Can you work these out from the model? Positions are in its coordinate system, mm. Face numbers are marked on the shaded views. A direction names the side the tool comes from. Give positions to 0.01 mm unless a question says otherwise; leave off trailing zeros. Write each loop counter-clockwise with the first axis right and the second up, starting at its lowest first coordinate (ties: lowest second). Pieces come first, ordered by that corner, then holes. Notation, with made-up numbers: (-29.5, -30) -> (-4.5, -30) arc R23 cw to (-4.5, 1) -> close; hole circle Ø7 at (-39, 73.25). An arc over 180 degrees is marked (long way). Answer as CSV lines item,"result". Start each with the question number.
1. If we mould it in two halves opening along Z, with no side actions, what happens to the marked faces 3, 4, 5 and 6? For each: pulls with the +Z half, pulls with the -Z half, needs draft (parallel to the pull), parting line crosses it, or undercut.
2. If we section it at C-C on x = 1.8: Write out the boundary of the cut face in (y, z), plus the area to 3 significant figures.
3. I need wall thicknesses on line 1 (Y direction, x = -0.9, z = 0); line 2 (X direction, y = 0.75, z = 2.5); line 3 (Y direction, x = 1.1, z = -0.75). Which ranges of each line are inside material? Lowest first, please. Write a range as [from, to].
4. If we section it at B-B on x = -1.9: Write out the boundary of the cut face in (y, z).
5. On a 3-axis mill with a long thin cutter (end or side, diameter ignored), from which of +Z, -Z, +X, -X, +Y, -Y can I reach the whole of each face in a straight line? I mean the marked faces 1 and 2. Say none if no direction works.
6. If we section it at A-A on z = 0: Write out the boundary of the cut face in (x, y).
7. I'm going to push flat-ended pins straight in: P1, Ø1.1, axis at x = 2, y = -2, coming from the -Z side; P2, Ø0.5, axis at x = 2, y = 0, coming from the +Z side; P3, Ø1, axis at x = -2.5, z = -1.5, coming from the -Y side. Where does each tip first touch, or does it pass through?
Autodesk Inventor part; units mm, degrees
ref_plane "YZ Plane" through (0, 0, 0) normal (1, 0, 0) x (0, 1, 0)
ref_plane "XZ Plane" through (0, 0, 0) normal (0, 1, 0) x (-1, 0, 0)
ref_plane "XY Plane" through (0, 0, 0) normal (0, 0, 1) x (1, 0, 0)
sketch "Sketch1" plane through (0, 0, 0) normal (1, 0, 0) x (0, 1, 0)
  circle A0 centre (0, 0) radius 5
  dimension "d0" = 5
extrude "Extrusion1" add sketch "Sketch1" along normal blind 2.6
fillet "Fillet1" radius 2 1 edges at (2.6, -5, 0)
sketch "Sketch2" plane through (2.6, 0, 0) normal (1, 0, 0) x (0, 0, -1)
  circle A0 centre (0, 0) radius 3
  circle A1 centre (0, 0) radius 5
  circle A2 centre (0, 0) radius 3
  circle A3 centre (0, 0) radius 5
  line L0 (1, 4.899) -> (1, -4.899)
  line L1 (-1, 4.899) -> (-1, -4.899)
  dimension "d4" = 1
  dimension "d5" = 1
extrude "Extrusion2" cut sketch "Sketch2" against normal blind 1 contours L0 A0 L1 | A0 L1 A1 L0 | L0 A1 L1 A0
sketch "Sketch3" plane through (0, 0, 0) normal (-1, 0, 0) x (0, 0, 1)
  circle A0 centre (0, 0) radius 2.5
  dimension "d8" = 2.5
extrude "Extrusion3" add sketch "Sketch3" along normal blind 3
sketch "Sketch4" plane through (-3, 0, 0) normal (-1, 0, 0) x (0, 0, 1)
  circle A0 centre (0, 0) radius 1
  dimension "d11" = 1
extrude "Extrusion4" cut sketch "Sketch4" against normal through all
properties part number "nutsert"
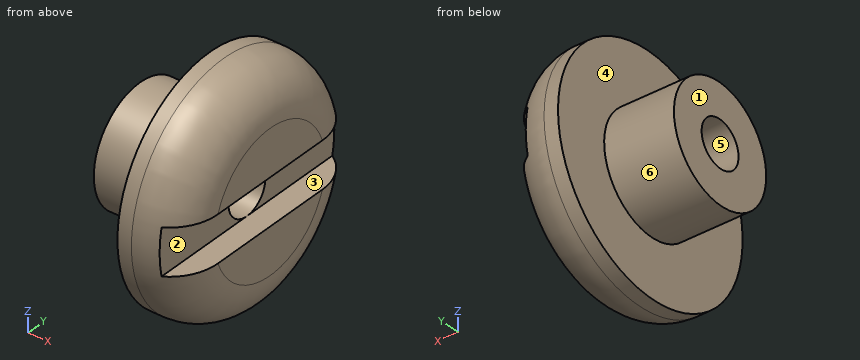
Computed values:
1,face 3,"undercut"
1,face 4,"needs draft"
1,face 5,"undercut"
1,face 6,"parting line crosses it"
2,outline,"(-4.49, -1) arc R4.6 ccw to (4.49, -1) -> close; (-4.49, 1) -> (4.49, 1) arc R4.6 ccw to start"
2,area,"48.2 mm2"
3,line 1,"y = [-2.5, -1], [1, 2.5]"
3,line 2,"x = [0, 2.6]"
3,line 3,"y = [-4.88, -0.66], [0.66, 4.88]"
4,outline,"circle Ø5 at (0, 0); hole circle Ø2 at (0, 0)"
5,face 1,"+Z, -Z, -X, +Y, -Y"
5,face 2,"+X, +Y, -Y"
6,outline,"(-3, -2.5) -> (0, -2.5) -> (0, -5) -> (0.6, -5) arc R2 ccw to (1.6, -4.73) -> (1.6, -1) -> (-3, -1) -> close; (-3, 1) -> (1.6, 1) -> (1.6, 4.73) arc R2 ccw to (0.6, 5) -> (0, 5) -> (0, 2.5) -> (-3, 2.5) -> close"
7,P1,"stops at z = -4.45"
7,P2,"stops at z = 4.64"
7,P3,"stops at y = -2.29"
